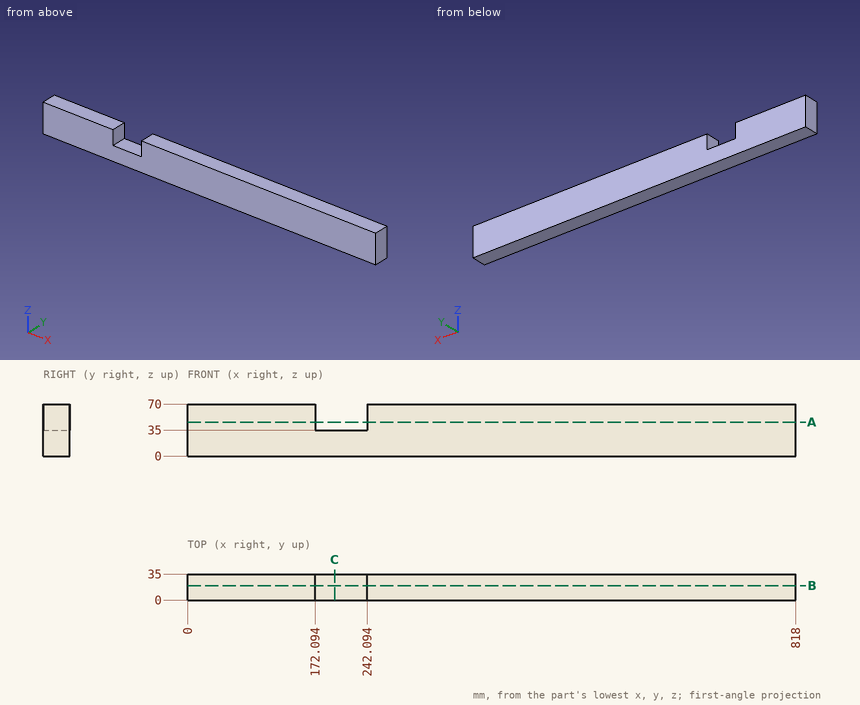
Could you check a few things on this drawing? It's one solid part, dimensions in mm from its lowest x, y, z. Give positions to 0.01 mm unless a question says otherwise; leave off trailing zeros. Write each loop counter-clockwise with the first axis right and the second up, starting at its lowest first coordinate (ties: lowest second). Pieces come first, ordered by that corner, then holes. Notation, with made-up numbers: (-28.75, 12.5) - (-20.75, 12.5) arc R20 ccw to (-20.75, 46.5) - close; hole circle Ø8 at (23.5, 37.25). An arc over 180 degrees is marked (long way). Use CSV: the item, a comma, the result in double quotes. Start each with the question number.
Item 1: If I drill on line 1 along X through (y, z) = (30.5, 36); line 2 along Z through (x, y) = (203, 8.5), over which ranges is the centre line in solid material (lowest first)?
Item 2: I want a section at A-A, the plane z = 45.5. Please give me the cut outline in (x, y).
Item 3: I want a section at C-C, the plane x = 198. Please give me the cut outline in (y, z), then the cut area to 4 significant figures.
Item 4: I want a section at B-B, the plane y = 19.5. Please give me the cut outline in (x, z).
Item 5: I'm going to push a flat-ended pin straight in: pin 1 (6 mm diameter, centred on x = 234.5, y = 7.5, fed in from +Z). Where does the tip first touch, or does it pass through?
Findings:
1,line 1,"x = 0 to 172.09, 242.09 to 818"
1,line 2,"z = 0 to 35"
2,outline,"(0, 0) - (172.09, 0) - (172.09, 35) - (0, 35) - close; (242.09, 0) - (818, 0) - (818, 35) - (242.09, 35) - close"
3,outline,"(0, 0) - (35, 0) - (35, 35) - (0, 35) - close"
3,area,"1,225 mm2"
4,outline,"(0, 0) - (818, 0) - (818, 70) - (242.09, 70) - (242.09, 35) - (172.09, 35) - (172.09, 70) - (0, 70) - close"
5,pin 1,"stops at z = 35"
